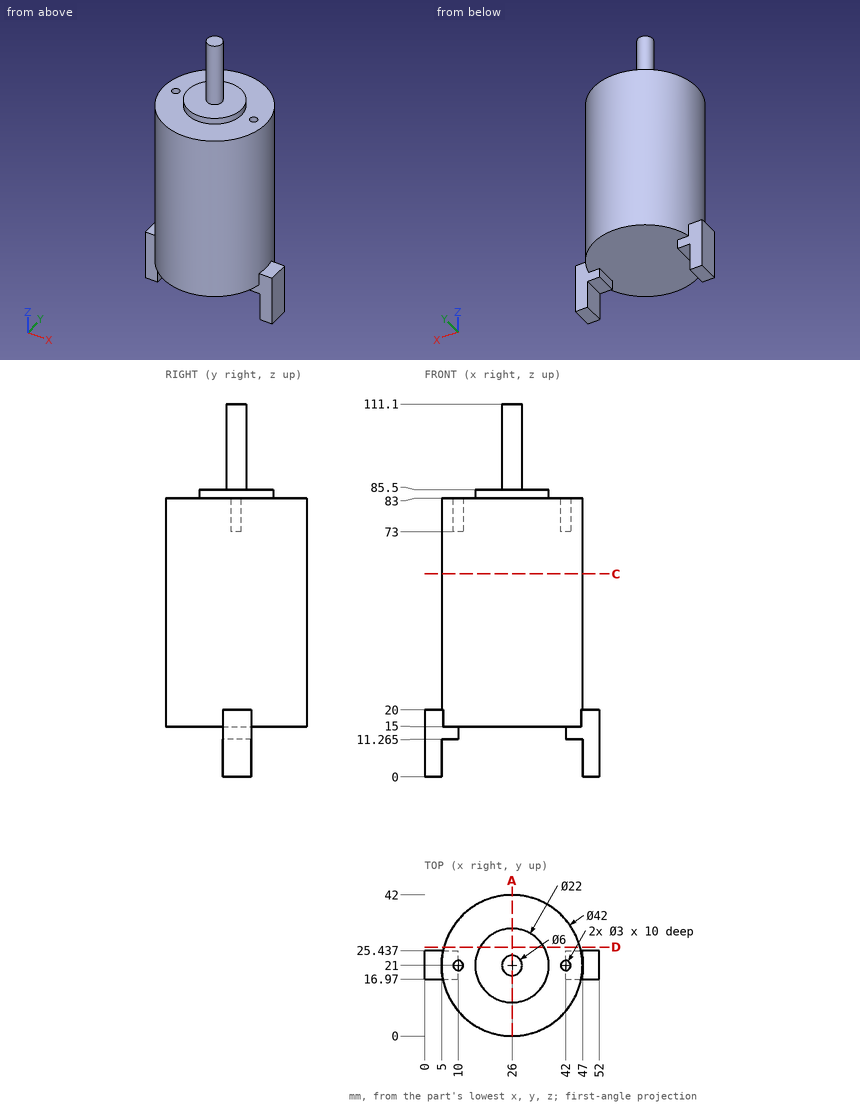
Study the drawing (mm; zero at the part's minimum x, y, z) and answer. Give positions to 0.01 mm unless a question says otherwise; leave off trailing zeros. Order: outer loops, then holes, each group sorted by start corner. A loop starts at its lowest first (then second) coordinate and runs counter-clockwise, first axis right, second up. Notation, with made-up numbers: M 65,-19.5 L 69,-19.5 A30 cw 69,19.5 Z; hole C -3.5,4 d9. An arc over 180 degrees is marked long. Put each result on its own line as item: value. Start each with the question number.
Item 1: The part is cut by section D-D, the plane y = 26.5. Determine the outline of the cut face in (x, z).
Item 2: Find the intervals of material crossed by line 1 along Z through (x, y) = (24, 8); line 2 along X through (y, z) = (18.5, 14.5); line 3 along Y through (x, z) = (10, 79), in increasing order.
Item 3: The part is cut by section C-C, the plane z = 60.5. Determine the outline of the cut face in (x, y), and give its area (3 significant figures).
Item 4: The part is cut by section A-A, the plane x = 26. Determine the outline of the cut face in (y, z).
Item 5: Flat-ended cylindrical pins translate along their axes: P1, Ø2.5, axis at x = 10, y = 21, coming from the +Z side; P2, Ø4, axis at x = 14.5, y = 11, coming from the -Z side; P3, Ø6, axis at x = 36, z = 60.5, coming from the -Y side; P4, Ø1.5, axis at x = 41.5, z = 84, coming from the -Y side. Find the tip coordinate at first contact, or state that the pin passes through.
Answer key:
1. outline: M 5.73,15 L 46.27,15 L 46.27,83 L 35.53,83 L 35.53,85.5 L 16.47,85.5 L 16.47,83 L 5.73,83 Z
2. line 1: z = 15 to 83
2. line 2: x = 0 to 10, 42 to 52
2. line 3: y = 7.4 to 19.5, 22.5 to 34.6
3. outline: C 26,21 d42
3. area: 1,390 mm²
4. outline: M 0,15 L 42,15 L 42,83 L 32,83 L 32,85.5 L 24,85.5 L 24,111.1 L 18,111.1 L 18,85.5 L 10,85.5 L 10,83 L 0,83 Z
5. P1: stops at z = 73
5. P2: stops at z = 15
5. P3: stops at y = 1.2
5. P4: passes through
